from build123d import *

# Parameters (mm, degrees)
SKETCH1_R                     = 7.5
BOSS_EXTRUDE1_DEPTH           = 15
BOSS_EXTRUDE1_TAPER           = 1
BOSS_EXTRUDE1_OTHER_WAY_DEPTH = 10
BOSS_EXTRUDE1_OTHER_WAY_TAPER = -1
CUT_EXTRUDE1_DEPTH            = 19.514790178
CUT_EXTRUDE1_DEPTH_BACK       = 19.514790178
CUT_EXTRUDE2_START            = -10.593003294
CUT_EXTRUDE2_OUTLINE_W        = 6.502745185
CUT_EXTRUDE2_OUTLINE_H        = 10
CUT_EXTRUDE2_DEPTH            = 10.593003294
SKETCH5_R                     = 1.5
CUT_EXTRUDE3_DEPTH            = 21.979721988
FILLET1_SIZE                  = 5
CUT_EXTRUDE4_DEPTH            = 19.443121582
CUT_EXTRUDE4_DEPTH_BACK       = 19.443121582
SKETCH6_W                     = 21.270993481
SKETCH6_H                     = 9.912737968
CUT_EXTRUDE5_DEPTH            = 19.514162399
SKETCH8_R                     = 1
CUT_EXTRUDE6_DEPTH            = 19.514162399
BOSS_EXTRUDE2_DEPTH           = 0.5


with BuildPart() as part:
    # Sketch1 → Boss-Extrude1 (new body)
    with BuildSketch(Plane(origin=(0, 0, 0), x_dir=(1, 0, 0), z_dir=(0, 1, 0))):
        Circle(SKETCH1_R)
    extrude(amount=BOSS_EXTRUDE1_DEPTH, taper=BOSS_EXTRUDE1_TAPER)

    # Sketch1 → Boss-Extrude1 other way (add)
    with BuildSketch(Plane(origin=(0, 0, 0), x_dir=(1, 0, 0), z_dir=(0, 1, 0))):
        Circle(SKETCH1_R)
    extrude(amount=-BOSS_EXTRUDE1_OTHER_WAY_DEPTH, taper=BOSS_EXTRUDE1_OTHER_WAY_TAPER)

    # Sketch3 → Cut-Extrude1 (cut, two sides: drawn at the far end of the back side and taken through both)
    with BuildSketch(Plane(origin=(0, 0, 0), x_dir=(0, 0, -1), z_dir=(1, 0, 0)).offset(-CUT_EXTRUDE1_DEPTH_BACK)):
        Polygon((-2.918452544, -10), (-2.918452544, 0), (-14.964340612, 6.954696718), (-14.964340612, -10), align=None)
    extrude(amount=CUT_EXTRUDE1_DEPTH + CUT_EXTRUDE1_DEPTH_BACK, mode=Mode.SUBTRACT)

    # Cut-Extrude2: read off the stored shape, not the designer's step
    # Cut-Extrude2 outline → Cut-Extrude2 (cut)
    with BuildSketch(Plane.XY.offset(2.918452544).offset(CUT_EXTRUDE2_START)):
        with Locations((-8.251372593, -5)):
            Rectangle(CUT_EXTRUDE2_OUTLINE_W, CUT_EXTRUDE2_OUTLINE_H)
        with Locations((8.251372593, -5)):
            Rectangle(CUT_EXTRUDE2_OUTLINE_W, CUT_EXTRUDE2_OUTLINE_H)
    extrude(amount=CUT_EXTRUDE2_DEPTH, mode=Mode.SUBTRACT)

    # Sketch5 → Cut-Extrude3 (cut, through all)
    with BuildSketch(Plane(origin=(5, 0, 0), x_dir=(0, 0, -1), z_dir=(1, 0, 0))):
        with Locations((1.081547456, -6)):
            Circle(SKETCH5_R)
    extrude(amount=-CUT_EXTRUDE3_DEPTH, mode=Mode.SUBTRACT)

    # Fillet1
    # a fillet whose section is not a circle: 5 mm, written as the material it takes off along each edge
    with BuildSketch(Plane(origin=(17.5, -10, 2.918452544), x_dir=(0, 0, -1), z_dir=(-1, 0, 0))) as fillet1_piece_1:
        with BuildLine():
            Bezier((FILLET1_SIZE, 0), (0, 0), (0, -FILLET1_SIZE), weights=[1, 1.5, 1])
            Line((0, -FILLET1_SIZE), (0, 0))
            Line((0, 0), (FILLET1_SIZE, 0))
        make_face()
    extrude(amount=35, mode=Mode.SUBTRACT)

    # Fillet2
    # a fillet whose section is not a circle: 10, 5 mm, written as the material it takes off along each edge
    with BuildSketch(Plane(origin=(0, 15, 0), x_dir=(1, 0, 0), z_dir=(0, 0, -1))) as fillet2_piece_1:
        with BuildLine():
            Bezier((7.411201511, 9.912737968), (7.238174026, 0), (2.411963035, 0), weights=[1, 0.818181818, 1])
            Line((2.411963035, 0), (7.238174026, 0))
            Line((7.238174026, 0), (7.411201511, 9.912737968))
        make_face()
    revolve(axis=Axis((0, 15, 0), (0, -1, 0)), mode=Mode.SUBTRACT)

    # Sketch6 → Cut-Extrude4 (cut, two sides: drawn at the far end of the back side and taken through both)
    with BuildSketch(Plane(origin=(0, 0, 0), x_dir=(0, 0, -1), z_dir=(1, 0, 0)).offset(-CUT_EXTRUDE4_DEPTH_BACK)):
        with Locations((-1.160829525, 10.043631016)):
            Rectangle(SKETCH6_W, SKETCH6_H)
    extrude(amount=CUT_EXTRUDE4_DEPTH + CUT_EXTRUDE4_DEPTH_BACK, mode=Mode.SUBTRACT)

    # Sketch7 → Cut-Extrude5 (cut, through all)
    with BuildSketch(Plane.XZ.offset(10)):
        with BuildLine():
            Line((4, -2.081547456), (4, -4.024987586))
            ThreePointArc((4, -4.024987586), (0, -5.674550649), (-4, -4.024987586))
            Line((-4, -4.024987586), (-4, -2.081547456))
            Line((-4, -2.081547456), (4, -2.081547456))
        make_face()
    extrude(amount=-CUT_EXTRUDE5_DEPTH, mode=Mode.SUBTRACT)

    # Sketch8 → Cut-Extrude6 (cut, through all)
    with BuildSketch(Plane(origin=(0, 5.087262032, 0), x_dir=(1, 0, 0), z_dir=(0, 1, 0))):
        with Locations(Location((0, -4, 0), (0, 0, 270))):
            Circle(SKETCH8_R)
    extrude(amount=-CUT_EXTRUDE6_DEPTH, mode=Mode.SUBTRACT)

    # Sketch9 → Cut-Revolve3 (revolve, cut)
    with BuildSketch(Plane(origin=(0, 5.087262032, 0), x_dir=(1, 0, 0), z_dir=(0, 1, 0))):
        with BuildLine():
            Line((-2, -0.30500636), (2, -0.30500636))
            ThreePointArc((2, -0.30500636), (0, 1.69499364), (-2, -0.30500636))
        make_face()
    revolve(axis=Axis((-2, 5.087262032, 0.30500636), (1, 0, 0)), mode=Mode.SUBTRACT)

    # Sketch10 → Boss-Extrude2 (add)
    with BuildSketch(Plane(origin=(0, 5.087262032, 0), x_dir=(1, 0, 0), z_dir=(0, 1, 0))):
        with BuildLine():
            Line((-1.936491673, -0.80500636), (1.936491673, -0.80500636))
            ThreePointArc((1.936491673, -0.80500636), (2, -0.30500636), (1.936491673, 0.19499364))
            Line((1.936491673, 0.19499364), (-1.936491673, 0.19499364))
            ThreePointArc((-1.936491673, 0.19499364), (-2, -0.30500636), (-1.936491673, -0.80500636))
        make_face()
    extrude(amount=-BOSS_EXTRUDE2_DEPTH)


solid = part.part
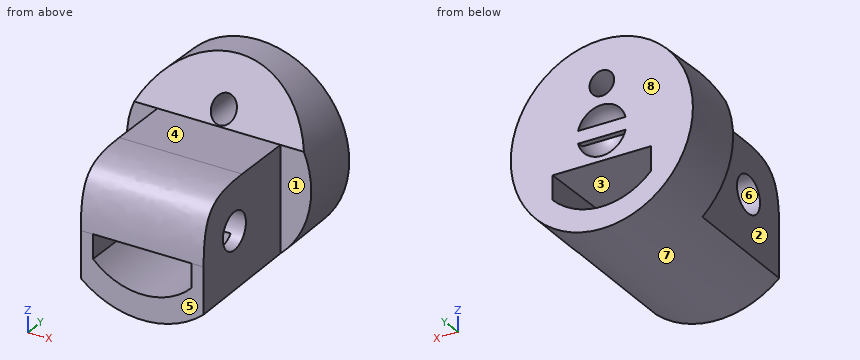
Read the model definition and answer for the solid it produces. Units are mm, in the model's axes. Face numbers are marked on the shaded views. A direction names the side the tool comes from. Give positions to 0.01 mm unless a question says otherwise; leave off trailing zeros. Write each loop counter-clockwise with the first axis right and the second up, starting at its lowest first coordinate (ties: lowest second). Pieces come first, ordered by that corner, then holes. Notation, with made-up numbers: (-5.5, 77) - (3.5, 77) arc R17 ccw to (3.5, 82) - close; hole circle Ø8 at (62, 31). An arc over 180 degrees is marked (long way). Answer in a Markdown table with one row per item. Add a question column.
Item 1: Section A-A, the plane y = -3.5 is taken. Write down the section's boundary in (x, z), and give its area (3 significant figures).
Item 2: Section B-B, the plane x = 0 is taken. Count the separate pieces of the cut face and the enclosed holes in it, and give its area (3 significant figures).
Item 3: A tool of negligible diameter and unlimited length cuts with its end or side. For the marked faces 1, 2, 3, 4 and 5, from which of +Z, -Z, +X, -X, +Y, -Y can it reach the whole face along a straight path? Write none if from no direction.
Item 4: Find the intervals of material crossed by L1, parallel to Z at x = 0, y = 2.9; L2, parallel to Y at x = -6, z = -2.5; L3, parallel to Z at x = 0, y = 1.7, in increasing order.
Item 5: Determine the mould class of the marked faces 6, 7 and 8 for opening direction Z: pulls with the +Z half, pulls with the -Z half, needs draft (parallel to the pull), parting line crosses it, or undercut.
Item 6: Flat-ended cylindrical pins translate along their axes: P1, Ø1.5, axis at x = 2, y = -2, coming from the +Z side; P2, Ø2, axis at y = -3.5, z = 4.5, coming from the +X side; P3, Ø1.6, axis at y = -3, z = -2.5, coming from the -X side; P4, Ø0.6, axis at x = 1, y = 5, coming from the +Z side. Find the tip coordinate at first contact, or state that the pin passes through.
Recorded:
| question | item | result |
|---|---|---|
| 1 | outline | (-5, -5.67) arc R7.56 ccw to (5, -5.67) - (5, 2.92) - (-5, 2.92) - close; hole (-4, -4.02) arc R5.67 ccw to (4, -4.02) - (4, -2.08) - (-4, -2.08) - close |
| 1 | area | 74.2 mm2 |
| 2 | separate pieces | 4 |
| 2 | enclosed holes | 0 |
| 2 | area | 96.8 mm2 |
| 3 | face 1 | +Z, -Z, +X, -Y |
| 3 | face 2 | +Z, -Z, -X, -Y |
| 3 | face 3 | +Y, -Y |
| 3 | face 4 | +Z, +X, -X, -Y |
| 3 | face 5 | +Z, -Z, +X, -X, -Y |
| 4 | L1 | z = -7.45 to -5.67, -2.08 to 3, 5 to 7.45 |
| 4 | L2 | y = 0 to 5.09 |
| 4 | L3 | z = -7.47 to -5.67, -2.08 to 3, 5 to 5.86 |
| 5 | face 6 | undercut |
| 5 | face 7 | parting line crosses it |
| 5 | face 8 | needs draft |
| 6 | P1 | stops at z = 2.92 |
| 6 | P2 | passes through |
| 6 | P3 | stops at x = -5 |
| 6 | P4 | stops at z = 7.38 |
